CAD build for the part. Positions are in the model's coordinates, mm. A direction names the side the tool comes from. Give positions to 0.01 mm unless a question says otherwise; leave off trailing zeros. Write each loop counter-clockwise with the first axis right and the second up, starting at its lowest first coordinate (ties: lowest second). Pieces come first, ordered by that corner, then holes. Notation, with made-up numbers: (30, 39) - (58, 39) arc R12 cw to (58, 46) - close; hole circle Ø8 at (37, 47). An arc over 180 degrees is marked (long way). Answer as a JSON object with one key per item and string values.
from build123d import *

# Parameters (mm, degrees)
Y_KSEKLIK_EKSTR_ZYON1_DEPTH = 12
KES_EKSTR_ZYON1_DEPTH       = 10
Y_KSEKLIK_EKSTR_ZYON7_DEPTH = 1
IZIM4_R                     = 1
KES_EKSTR_ZYON2_DEPTH       = 11
IZIM6_R                     = 4.25
KES_EKSTR_ZYON3_DEPTH       = 1.5


with BuildPart() as part:
    # Çizim1 → Yükseklik-Ekstrüzyon1 (new body)
    with BuildSketch(Plane.XY):
        with BuildLine():
            ThreePointArc((3.192280857, -0.60978925), (2.975857359, -1.065220637), (2.56471968, -1.357149888))
            ThreePointArc((2.56471968, -1.357149888), (2.234721924, -2.513666231), (3.437313781, -2.499474739))
            ThreePointArc((3.437313781, -2.499474739), (4.19799408, 0.662831579), (2.5, 3.436931771))
            Line((2.5, 3.436931771), (2.5, 8.97649343))
            ThreePointArc((2.5, 8.97649343), (1.914213562, 10.390706993), (0.5, 10.97649343))
            Line((0.5, 10.97649343), (-0.5, 10.97649343))
            ThreePointArc((-0.5, 10.97649343), (-1.914213562, 10.390706993), (-2.5, 8.97649343))
            Line((-2.5, 8.97649343), (-2.5, 3.436931771))
            ThreePointArc((-2.5, 3.436931771), (-4.25, 0), (-2.5, -3.436931771))
            Line((-2.5, -3.436931771), (-2.5, -8.97649343))
            ThreePointArc((-2.5, -8.97649343), (-1.914213562, -10.390706993), (-0.5, -10.97649343))
            Line((-0.5, -10.97649343), (0.5, -10.97649343))
            ThreePointArc((0.5, -10.97649343), (1.914213562, -10.390706993), (2.5, -8.97649343))
            Line((2.5, -8.97649343), (2.5, -3.534499959))
            ThreePointArc((2.5, -3.534499959), (2.485291154, -3.44171549), (2.442606949, -3.35802937))
            Line((2.442606949, -3.35802937), (2.429810536, -3.340437211))
            ThreePointArc((2.429810536, -3.340437211), (1.892940792, -2.966324418), (1.239680541, -3.004278975))
            ThreePointArc((1.239680541, -3.004278975), (-2.518723033, 2.053907077), (3.192280857, -0.60978925))
        make_face()
        with BuildLine():
            Line((1.5, 3.97649343), (1.5, 8.97649343))
            ThreePointArc((1.5, 8.97649343), (1.207106781, 9.683600211), (0.5, 9.97649343))
            Line((0.5, 9.97649343), (-0.5, 9.97649343))
            ThreePointArc((-0.5, 9.97649343), (-1.207106781, 9.683600211), (-1.5, 8.97649343))
            Line((-1.5, 8.97649343), (-1.5, 3.97649343))
            ThreePointArc((-1.5, 3.97649343), (0, 4.25), (1.5, 3.97649343))
        make_face(mode=Mode.SUBTRACT)
        with BuildLine():
            ThreePointArc((0.5, -9.97649343), (1.207106781, -9.683600211), (1.5, -8.97649343))
            Line((1.5, -8.97649343), (1.5, -3.97649343))
            ThreePointArc((1.5, -3.97649343), (0, -4.25), (-1.5, -3.97649343))
            Line((-1.5, -3.97649343), (-1.5, -8.97649343))
            ThreePointArc((-1.5, -8.97649343), (-1.207106781, -9.683600211), (-0.5, -9.97649343))
            Line((-0.5, -9.97649343), (0.5, -9.97649343))
        make_face(mode=Mode.SUBTRACT)
    extrude(amount=Y_KSEKLIK_EKSTR_ZYON1_DEPTH)

    # Çizim2 → Kes-Ekstrüzyon1 (cut)
    with BuildSketch(Plane.XY.offset(12)):
        with BuildLine():
            Line((-2.5, -3.436931771), (-2.5, -10.97649343))
            Line((-2.5, -10.97649343), (2.5, -10.97649343))
            Line((2.5, -10.97649343), (2.5, -3.436931771))
            ThreePointArc((2.5, -3.436931771), (0, -4.25), (-2.5, -3.436931771))
        make_face()
    extrude(amount=-KES_EKSTR_ZYON1_DEPTH, mode=Mode.SUBTRACT)

    # Çizim3 → Yükseklik-Ekstrüzyon7 (add)
    with BuildSketch(Plane(origin=(0, 0, 0), x_dir=(-1, 0, 0), z_dir=(0, 0, -1))):
        with BuildLine():
            ThreePointArc((-2.5, 11.97649343), (-1.914213562, 13.390706993), (-0.5, 13.97649343))
            Line((-0.5, 13.97649343), (0.5, 13.97649343))
            ThreePointArc((0.5, 13.97649343), (1.914213562, 13.390706993), (2.5, 11.97649343))
            Line((2.5, 11.97649343), (2.5, 8.97649343))
            ThreePointArc((2.5, 8.97649343), (1.914213562, 10.390706993), (0.5, 10.97649343))
            Line((0.5, 10.97649343), (-0.5, 10.97649343))
            ThreePointArc((-0.5, 10.97649343), (-1.914213562, 10.390706993), (-2.5, 8.97649343))
            Line((-2.5, 8.97649343), (-2.5, 11.97649343))
        make_face()
    extrude(amount=-Y_KSEKLIK_EKSTR_ZYON7_DEPTH)

    # Çizim4 → Kes-Ekstrüzyon2 (cut)
    with BuildSketch(Plane(origin=(0, 0, 0), x_dir=(-1, 0, 0), z_dir=(0, 0, -1))):
        with Locations((0, 11.97649343)):
            Circle(IZIM4_R)
    extrude(amount=-KES_EKSTR_ZYON2_DEPTH, mode=Mode.SUBTRACT)

    # Çizim6 → Kes-Ekstrüzyon3 (cut)
    with BuildSketch(Plane.XY.offset(12)):
        Circle(IZIM6_R)
    extrude(amount=-KES_EKSTR_ZYON3_DEPTH, mode=Mode.SUBTRACT)


solid = part.part
(1) 3-axis set-ups, long thin cutter, end or side, ignore diameter. For faces 1 (the face through (-1.21, -9.68, 0.99)), 2 (the face through (-2, 7, 12)), 3 (the face through (-2.5, -6, 1)), 4 (the face through (-2.011, 3.744, 11.26)), 5 (the face through (-1.899, 10.406, 6.423)): which of +Z, -Z, +X, -X, +Y, -Y reach the whole face in a straight line?
Answer key:
{"face 1": "+Z, -Z", "face 2": "+Z, +X, -X, +Y, -Y", "face 3": "+Z, -Z, -X, -Y", "face 4": "+Z, -Y", "face 5": "+Z, -X, +Y"}
(2) Saw through at C-C, the plane y = 8.25. Give the cut face in (x, z), and give its area (3 significant figures).
Answer key:
{"outline": "(-2.5, 0) - (-1.5, 0) - (-1.5, 12) - (-2.5, 12) - close; (1.5, 0) - (2.5, 0) - (2.5, 12) - (1.5, 12) - close", "area": "24.0 mm²"}
(3) Flat gauge pins, fed straight in: P1, Ø1.5, axis at y = 5.5, z = 8, coming from the +X side; P2, Ø0.5, axis at x = 0, z = 4.5, coming from the +Y side; P3, Ø1.6, axis at y = -7, z = 0.5, coming from the -X side; P4, Ø5, axis at x = 2.5, y = -3.5, coming from the -Z side. Where does each tip first touch, or does it go through?
Answer key:
{"P1": "stops at x = 2.5", "P2": "stops at y = 10.98", "P3": "stops at x = -2.5", "P4": "stops at z = 0"}
(4) Saw through at A-A, the plane y = -6.25. Give the cut face in (x, z), and give its area (3 significant figures).
Answer key:
{"outline": "(-2.5, 0) - (-1.5, 0) - (-1.5, 2) - (-2.5, 2) - close; (1.5, 0) - (2.5, 0) - (2.5, 2) - (1.5, 2) - close", "area": "4.00 mm²"}
(5) Probe L1, parallel to Y at x = 0, z = 5; L2, parallel to Y at x = 0, z = 0.8; L3, parallel to X at y = 8.25, z = 10.75. List the from-to ranges inside material, lowest first. Write a range as [from, to].
Answer key:
{"L1": "y = [-4.25, -3.25], [3.25, 4.25], [9.98, 10.98]", "L2": "y = [-10.98, -9.98], [-4.25, -3.25], [3.25, 4.25], [9.98, 10.98], [12.98, 13.98]", "L3": "x = [-2.5, -1.5], [1.5, 2.5]"}
